For this review, take the finished solid that the model builds, in its own axes (mm). A direction names the side the tool comes from. Give positions to 0.01 mm unless a question says otherwise; leave off trailing zeros. Loops run counter-clockwise (first coordinate to the right, second up) from the corner with the lowest first, then second, coordinate; pieces in that order, holes last.
```python
from build123d import *

# Parameters (mm, degrees)
SKETCH_1_W          = 20
SKETCH_1_H          = 20
SKETCH_1_R          = 6.2
SKETCH_1_W_2        = 15
SKETCH_1_H_2        = 10
SKETCH_1_W_3        = 10
SKETCH_1_H_3        = 15
EXTRUDE_1_DEPTH     = 5
SKETCH_2_R          = 1.25
CUT_EXTRUDE_1_DEPTH = 36.707142143
SKETCH_2_3_R        = 2
SKETCH_2_3_R_2      = 1.25
CUT_EXTRUDE_2_DEPTH = 3.5


with BuildPart() as part:
    # 草图1 → 凸台-拉伸1 (new body)
    # profile 1 of 5: a face of its own
    with BuildSketch(Plane(origin=(0, 0, 0), x_dir=(1, 0, 0), z_dir=(0, 1, 0))):
        Rectangle(SKETCH_1_W, SKETCH_1_H)
        with Locations(Location((0, 0, 0), (0, 0, 270))):
            Circle(SKETCH_1_R, mode=Mode.SUBTRACT)
    # profile 2 of 5: a face of its own
    with BuildSketch(Plane(origin=(0, 0, 0), x_dir=(1, 0, 0), z_dir=(0, 1, 0))):
        with Locations((-17.5, 0)):
            Rectangle(SKETCH_1_W_2, SKETCH_1_H_2)
    # profile 3 of 5: a face of its own
    with BuildSketch(Plane(origin=(0, 0, 0), x_dir=(1, 0, 0), z_dir=(0, 1, 0))):
        with Locations((0, -17.5)):
            Rectangle(SKETCH_1_W_3, SKETCH_1_H_3)
    # profile 4 of 5: a face of its own
    with BuildSketch(Plane(origin=(0, 0, 0), x_dir=(1, 0, 0), z_dir=(0, 1, 0))):
        with Locations((0, 17.5)):
            Rectangle(SKETCH_1_W_3, SKETCH_1_H_3)
    # profile 5 of 5: a face of its own
    with BuildSketch(Plane(origin=(0, 0, 0), x_dir=(1, 0, 0), z_dir=(0, 1, 0))):
        with Locations((17.5, 0)):
            Rectangle(SKETCH_1_W_2, SKETCH_1_H_2)
    extrude(amount=EXTRUDE_1_DEPTH)

    # 草图2 → 切除-拉伸1 (cut, through all)
    with BuildSketch(Plane.XZ):
        with Locations(Location((7, 7, 0), (0, 0, 270))):
            Circle(SKETCH_2_R)
        with Locations(Location((7, -7, 0), (0, 0, 270))):
            Circle(SKETCH_2_R)
        with Locations(Location((-7, -7, 0), (0, 0, 270))):
            Circle(SKETCH_2_R)
        with Locations(Location((-7, 7, 0), (0, 0, 270))):
            Circle(SKETCH_2_R)
        with Locations(Location((0, 21, 0), (0, 0, 270))):
            Circle(SKETCH_2_R)
        with Locations(Location((21, 0, 0), (0, 0, 270))):
            Circle(SKETCH_2_R)
        with Locations(Location((0, -21, 0), (0, 0, 270))):
            Circle(SKETCH_2_R)
        with Locations(Location((-21, 0, 0), (0, 0, 270))):
            Circle(SKETCH_2_R)
    extrude(amount=-CUT_EXTRUDE_1_DEPTH, mode=Mode.SUBTRACT)

    # 草图2<3> → 切除-拉伸2 (cut)
    # profile 1 of 8: a face of its own
    with BuildSketch(Plane.XZ):
        with Locations(Location((7, 7, 0), (0, 0, 270))):
            Circle(SKETCH_2_3_R)
        with Locations(Location((7, 7, 0), (0, 0, 270))):
            Circle(SKETCH_2_3_R_2, mode=Mode.SUBTRACT)
    # profile 2 of 8: a face of its own
    with BuildSketch(Plane.XZ):
        with Locations(Location((7, -7, 0), (0, 0, 270))):
            Circle(SKETCH_2_3_R)
        with Locations(Location((7, -7, 0), (0, 0, 270))):
            Circle(SKETCH_2_3_R_2, mode=Mode.SUBTRACT)
    # profile 3 of 8: a face of its own
    with BuildSketch(Plane.XZ):
        with Locations(Location((-7, 7, 0), (0, 0, 270))):
            Circle(SKETCH_2_3_R)
        with Locations(Location((-7, 7, 0), (0, 0, 270))):
            Circle(SKETCH_2_3_R_2, mode=Mode.SUBTRACT)
    # profile 4 of 8: a face of its own
    with BuildSketch(Plane.XZ):
        with Locations(Location((-7, -7, 0), (0, 0, 270))):
            Circle(SKETCH_2_3_R)
        with Locations(Location((-7, -7, 0), (0, 0, 270))):
            Circle(SKETCH_2_3_R_2, mode=Mode.SUBTRACT)
    # profile 5 of 8: a face of its own
    with BuildSketch(Plane.XZ):
        with Locations(Location((0, 21, 0), (0, 0, 270))):
            Circle(SKETCH_2_3_R)
        with Locations(Location((0, 21, 0), (0, 0, 270))):
            Circle(SKETCH_2_3_R_2, mode=Mode.SUBTRACT)
    # profile 6 of 8: a face of its own
    with BuildSketch(Plane.XZ):
        with Locations(Location((21, 0, 0), (0, 0, 270))):
            Circle(SKETCH_2_3_R)
        with Locations(Location((21, 0, 0), (0, 0, 270))):
            Circle(SKETCH_2_3_R_2, mode=Mode.SUBTRACT)
    # profile 7 of 8: a face of its own
    with BuildSketch(Plane.XZ):
        with Locations(Location((0, -21, 0), (0, 0, 270))):
            Circle(SKETCH_2_3_R)
        with Locations(Location((0, -21, 0), (0, 0, 270))):
            Circle(SKETCH_2_3_R_2, mode=Mode.SUBTRACT)
    # profile 8 of 8: a face of its own
    with BuildSketch(Plane.XZ):
        with Locations(Location((-21, 0, 0), (0, 0, 270))):
            Circle(SKETCH_2_3_R)
        with Locations(Location((-21, 0, 0), (0, 0, 270))):
            Circle(SKETCH_2_3_R_2, mode=Mode.SUBTRACT)
    extrude(amount=-CUT_EXTRUDE_2_DEPTH, mode=Mode.SUBTRACT)


solid = part.part
```
Q1. Consider section B-B on z = -21. Give the boundary of the cut face in (x, y).
Answers:
outline: (-5, 0) - (-2, 0) - (-2, 3.5) - (-1.25, 3.5) - (-1.25, 5) - (-5, 5) - close; (1.25, 3.5) - (2, 3.5) - (2, 0) - (5, 0) - (5, 5) - (1.25, 5) - close
Q2. Machinability: for faces 5 (the cylindrical face through (-7.76, 4.24, 7.99)), 6 (the flat face through (-6, 5, 4)), 7 (the flat face through (-10, 2, 8)), 8 (the flat face through (17, 2, 5)), 9 (the flat face through (-8, 3.5, 8)), which of the approach directions +Z, -Z, +X, -X, +Y, -Y give a long, thin tool a straight path to every point of the face, cutting with its end or side? Answer none if there is none.
Answers:
face 5: +Y, -Y
face 6: +Z, -Z, +X, -X, +Y
face 7: +Z, -X, +Y, -Y
face 8: +Z, +X, +Y, -Y
face 9: -Y
Q3. Consider section A-A on x = -7. Give the boundary of the cut face in (y, z).
Answers:
outline: (0, -10) - (5, -10) - (5, -8.25) - (3.5, -8.25) - (3.5, -9) - (0, -9) - close; (0, -5) - (3.5, -5) - (3.5, -5.75) - (5, -5.75) - (5, 5.75) - (3.5, 5.75) - (3.5, 5) - (0, 5) - close; (0, 9) - (3.5, 9) - (3.5, 8.25) - (5, 8.25) - (5, 10) - (0, 10) - close
Q4. Consider section C-C on y = 2.3. Count the separate pieces of the cut face and the enclosed holes in it, plus the area to 3 significant figures.
Answers:
separate pieces: 1
enclosed holes: 9
area: 779 mm2
Q5. For pin 1 Ø1 at (y, z) = (2.5, 8.5) entering from +X; pin 2 Ø3 at (x, z) = (0.5, -20.5) entering from -Y; pin 3 Ø1.5 at (x, y) = (-9, 2.5) entering from -Z; pin 4 Ø2.5 at (y, z) = (1.5, 7.5) entering from -X, all flat-tipped, find the tip position at first contact; note any pin that passes through.
Answers:
pin 1: stops at x = 10
pin 2: stops at y = 0
pin 3: stops at z = -10
pin 4: stops at x = -10
Q6. For probe 1 along X at (y, z) = (3.95, 0); probe 2 along X at (y, z) = (1.25, -7); probe 3 along X at (y, z) = (4.4, 21), list the stretches that pass through material, from the lowest coordinate up.
Answers:
probe 1: x = -25 to -22.25, -19.75 to -6.2, 6.2 to 19.75, 22.25 to 25
probe 2: x = -10 to -9, -5 to 5, 9 to 10
probe 3: x = -5 to -1.25, 1.25 to 5
Q7. Consider section D-D on x = -21. Give the boundary of the cut face in (y, z).
Answers:
outline: (0, -5) - (5, -5) - (5, -1.25) - (3.5, -1.25) - (3.5, -2) - (0, -2) - close; (0, 2) - (3.5, 2) - (3.5, 1.25) - (5, 1.25) - (5, 5) - (0, 5) - close
Q8. Mouldability with a two-part tool opening along Z and no side actions: class faces 1 (the cylindrical face through (-0.479, 4.24, 19.845)), 2 (the flat face through (-18, 2, -5)), 3 (the flat face through (-10, 2, -7)), 4 (the flat face through (1, 3.5, 20)) as +Z half, -Z half, draft (parallel to the pull), parting line (faces both ways), or undercut.
Answers:
face 1: undercut
face 2: -Z half
face 3: draft
face 4: undercut
